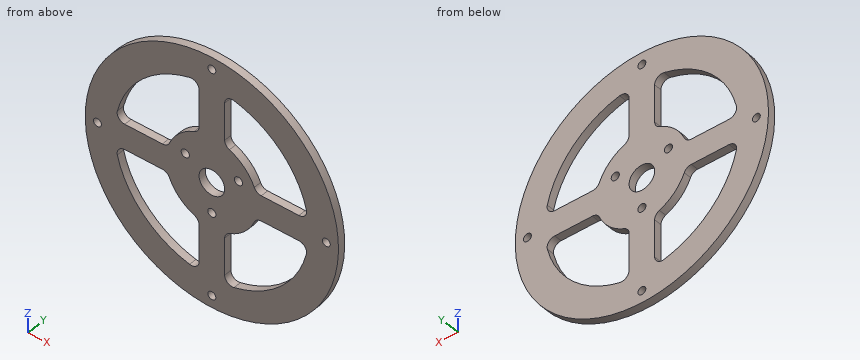
```python
from build123d import *

# Parameters (mm, degrees)
SKETCH_1_R      = 49.5
SKETCH_1_R_2    = 1.55
SKETCH_1_R_3    = 5
SKETCH_1_R_4    = 1.6
EXTRUDE_1_DEPTH = 3


with BuildPart() as part:
    # 草图1 → 凸台-拉伸1 (new body)
    with BuildSketch(Plane(origin=(0, 0, 0), x_dir=(1, 0, 0), z_dir=(0, 1, 0))):
        with Locations(Location((0, 0, 0), (0, 0, 270))):
            Circle(SKETCH_1_R)
        with Locations(Location((0, 44.75, 0), (0, 0, 270))):
            Circle(SKETCH_1_R_2, mode=Mode.SUBTRACT)
        with Locations(Location((-44.75, 0, 0), (0, 0, 270))):
            Circle(SKETCH_1_R_2, mode=Mode.SUBTRACT)
        with Locations(Location((0, -44.75, 0), (0, 0, 90))):
            Circle(SKETCH_1_R_2, mode=Mode.SUBTRACT)
        with Locations(Location((44.75, 0, 0), (0, 0, 90))):
            Circle(SKETCH_1_R_2, mode=Mode.SUBTRACT)
        with Locations(Location((0, 0, 0), (0, 0, 270))):
            Circle(SKETCH_1_R_3, mode=Mode.SUBTRACT)
        with Locations(Location((0, 12, 0), (0, 0, 270))):
            Circle(SKETCH_1_R_4, mode=Mode.SUBTRACT)
        with Locations(Location((10.392304845, -6, 0), (0, 0, 270))):
            Circle(SKETCH_1_R_4, mode=Mode.SUBTRACT)
        with Locations(Location((-10.392304845, -6, 0), (0, 0, 270))):
            Circle(SKETCH_1_R_4, mode=Mode.SUBTRACT)
        with BuildLine():
            Line((-34.045948677, 5), (-19.355269263, 5))
            ThreePointArc((-19.355269263, 5), (-17.687611546, 5.506224201), (-16.582759625, 6.854054841))
            ThreePointArc((-16.582759625, 6.854054841), (-12.687907325, 12.687907325), (-6.854054841, 16.582759625))
            ThreePointArc((-6.854054841, 16.582759625), (-5.506224201, 17.687611546), (-5, 19.355269263))
            Line((-5, 19.355269263), (-5, 34.045948677))
            ThreePointArc((-5, 34.045948677), (-6.137034306, 36.397407548), (-8.686239215, 36.966406815))
            ThreePointArc((-8.686239215, 36.966406815), (-26.851126462, 26.851126462), (-36.966406815, 8.686239215))
            ThreePointArc((-36.966406815, 8.686239215), (-36.397407548, 6.137034306), (-34.045948677, 5))
        make_face(mode=Mode.SUBTRACT)
        with BuildLine():
            Line((34.045948677, 5), (19.355269263, 5))
            ThreePointArc((19.355269263, 5), (17.687611546, 5.506224201), (16.582759625, 6.854054841))
            ThreePointArc((16.582759625, 6.854054841), (12.687907325, 12.687907325), (6.854054841, 16.582759625))
            ThreePointArc((6.854054841, 16.582759625), (5.506224201, 17.687611546), (5, 19.355269263))
            Line((5, 19.355269263), (5, 34.045948677))
            ThreePointArc((5, 34.045948677), (6.137034306, 36.397407548), (8.686239215, 36.966406815))
            ThreePointArc((8.686239215, 36.966406815), (26.851126462, 26.851126462), (36.966406815, 8.686239215))
            ThreePointArc((36.966406815, 8.686239215), (36.397407548, 6.137034306), (34.045948677, 5))
        make_face(mode=Mode.SUBTRACT)
        with BuildLine():
            Line((34.045948677, -5), (19.355269263, -5))
            ThreePointArc((19.355269263, -5), (17.687611546, -5.506224201), (16.582759625, -6.854054841))
            ThreePointArc((16.582759625, -6.854054841), (12.687907325, -12.687907325), (6.854054841, -16.582759625))
            ThreePointArc((6.854054841, -16.582759625), (5.506224201, -17.687611546), (5, -19.355269263))
            Line((5, -19.355269263), (5, -34.045948677))
            ThreePointArc((5, -34.045948677), (6.137034306, -36.397407548), (8.686239215, -36.966406815))
            ThreePointArc((8.686239215, -36.966406815), (26.851126462, -26.851126462), (36.966406815, -8.686239215))
            ThreePointArc((36.966406815, -8.686239215), (36.397407548, -6.137034306), (34.045948677, -5))
        make_face(mode=Mode.SUBTRACT)
        with BuildLine():
            Line((-34.045948677, -5), (-19.355269263, -5))
            ThreePointArc((-19.355269263, -5), (-17.687611546, -5.506224201), (-16.582759625, -6.854054841))
            ThreePointArc((-16.582759625, -6.854054841), (-12.687907325, -12.687907325), (-6.854054841, -16.582759625))
            ThreePointArc((-6.854054841, -16.582759625), (-5.506224201, -17.687611546), (-5, -19.355269263))
            Line((-5, -19.355269263), (-5, -34.045948677))
            ThreePointArc((-5, -34.045948677), (-6.137034306, -36.397407548), (-8.686239215, -36.966406815))
            ThreePointArc((-8.686239215, -36.966406815), (-26.851126462, -26.851126462), (-36.966406815, -8.686239215))
            ThreePointArc((-36.966406815, -8.686239215), (-36.397407548, -6.137034306), (-34.045948677, -5))
        make_face(mode=Mode.SUBTRACT)
    extrude(amount=EXTRUDE_1_DEPTH)


solid = part.part
```
The listing builds one solid part. Answer for the finished solid, in the listing's coordinates (mm). Round coordinates to 2 decimals unless told otherwise and drop trailing zeros. Order: outer loops, then holes, each group sorted by start corner. A loop starts at its lowest first (then second) coordinate and runs counter-clockwise, first axis right, second up. Notation, with made-up numbers: (-33.5, 59) -> (11.5, 59) arc R24 ccw to (11.5, 94) -> close; hole circle Ø10 at (20, -32). An arc over 180 degrees is marked (long way). Answer as CSV lines item,"result".
Q1. A cutting plane is placed at B-B on z = 35.5. Determine the outline of the cut face in (x, y), plus the area to 3 significant figures.
Computed values:
outline,"(-34.5, 0) -> (-13.48, 0) -> (-13.48, 3) -> (-34.5, 3) -> close; (-5.38, 0) -> (5.38, 0) -> (5.38, 3) -> (-5.38, 3) -> close; (13.48, 0) -> (34.5, 0) -> (34.5, 3) -> (13.48, 3) -> close"
area,"158 mm^2"
Q2. Consider line 1 (X direction, y = 0.7, z = 0); line 2 (Z direction, x = 32.5, y = 1.1); line 3 (X direction, y = 2.7, z = 8). Determine where each line is inside the solid, lowest interval first. Write a range as from..to.
Computed values:
line 1,"x = -49.5..-46.3, -43.2..-5, 5..43.2, 46.3..49.5"
line 2,"z = -37.34..-19.64, -5..5, 19.64..37.34"
line 3,"x = -48.85..-37.05, -16.06..16.06, 37.05..48.85"
Q3. Given pin 1 (0.9 mm diameter, centred on x = -23, y = 1.5, fed in from -Z); pin 2 (3 mm diameter, centred on x = 44.75, z = 0, fed in from +Y); pin 3 (1 mm diameter, centred on x = -29, y = 1, fed in from +Z); pin 4 (0.9 mm diameter, centred on y = 1, z = 24.5, fed in from +X), each flat-ended and moving along its own axis, determine where each tip first touches the part or whether it passes through.
Computed values:
pin 1,"stops at z = -44.07"
pin 2,"passes through"
pin 3,"stops at z = 40.47"
pin 4,"stops at x = 43.26"
Q4. A cutting plane is placed at A-A on x = 0. Determine the outline of the cut face in (y, z), plus the area to 3 significant figures.
Computed values:
outline,"(0, -49.5) -> (3, -49.5) -> (3, -46.3) -> (0, -46.3) -> close; (0, -43.2) -> (3, -43.2) -> (3, -13.6) -> (0, -13.6) -> close; (0, -10.4) -> (3, -10.4) -> (3, -5) -> (0, -5) -> close; (0, 5) -> (3, 5) -> (3, 43.2) -> (0, 43.2) -> close; (0, 46.3) -> (3, 46.3) -> (3, 49.5) -> (0, 49.5) -> close"
area,"239 mm^2"
Q5. A cutting plane is placed at D-D on x = -44.75. Determine the outline of the cut face in (y, z).
Computed values:
outline,"(0, -21.16) -> (3, -21.16) -> (3, -1.55) -> (0, -1.55) -> close; (0, 1.55) -> (3, 1.55) -> (3, 21.16) -> (0, 21.16) -> close"
Q6. A cutting plane is placed at C-C on x = -32. Determine the outline of the cut face in (y, z).
Computed values:
outline,"(0, -37.77) -> (3, -37.77) -> (3, -20.44) -> (0, -20.44) -> close; (0, -5) -> (3, -5) -> (3, 5) -> (0, 5) -> close; (0, 20.44) -> (3, 20.44) -> (3, 37.77) -> (0, 37.77) -> close"
